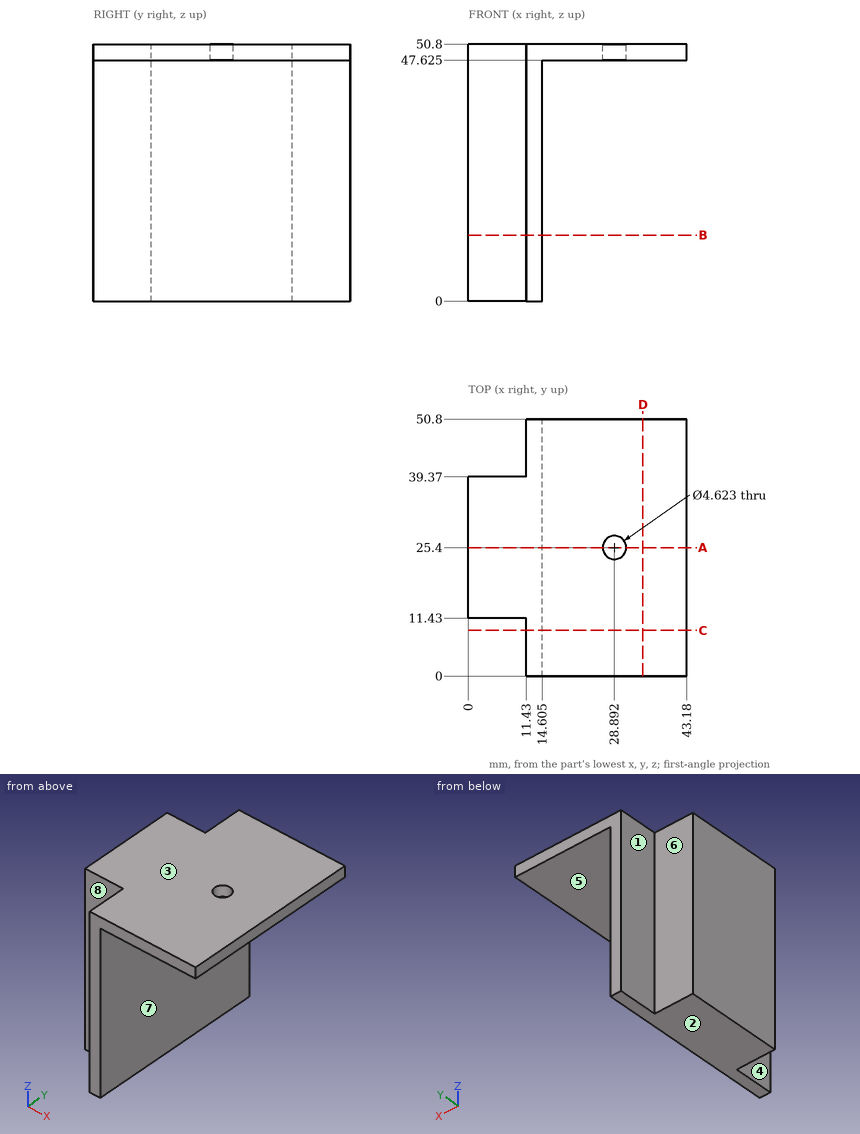
Job drawing, mm, ordinate dimensions from the low corner. One solid piece. A direction names the side the tool comes from. Round coordinates to 2 decimals unless told otherwise and drop trailing zeros. Loops run counter-clockwise (first coordinate to the right, second up) from the corner with the lowest first, then second, coordinate; pieces in that order, holes last. Notation, with made-up numbers: (85, -2) -> (142, -2) arc R22 ccw to (142, 16) -> close; hole circle Ø2 at (-7.75, 9.25). An arc over 180 degrees is marked (long way). Use a Markdown table: item, result.
1) Cut at B-B, the plane z = 13. List the corners of the cut face in (x, y) (1 decimal), and give its area (3 significant figures).
The answers:
| item | result |
|---|---|
| outline | (0, 11.4) -> (11.4, 11.4) -> (11.4, 0) -> (14.6, 0) -> (14.6, 50.8) -> (11.4, 50.8) -> (11.4, 39.4) -> (0, 39.4) -> close |
| area | 481 mm2 |
2) Pull direction Y, two halves, no side cores. Call the marked faces 6, 7 and 8: pulls with the +Y half, pulls with the -Y half, needs draft (parallel to the pull), parting line crosses it, or undercut.
The answers:
| item | result |
|---|---|
| face 6 | pulls with the +Y half |
| face 7 | needs draft |
| face 8 | pulls with the -Y half |
3) Cut at D-D, the plane x = 34.5. List the corners of the cut face in (y, z) (1 decimal), and give its area (3 significant figures).
The answers:
| item | result |
|---|---|
| outline | (0, 47.6) -> (50.8, 47.6) -> (50.8, 50.8) -> (0, 50.8) -> close |
| area | 161 mm2 |
4) Tool access for the marked faces 1, 2, 3, 4 and 5: list every direction of +Z, -Z, +X, -X, +Y, -Y with a clear straight run to the whole face (end or side of a thin tool).
The answers:
| item | result |
|---|---|
| face 1 | +Z, -Z, -X, +Y |
| face 2 | -Z, +X, -X, +Y, -Y |
| face 3 | +Z, +X, -X, +Y, -Y |
| face 4 | +Z, -Z, -X, -Y |
| face 5 | -Z, +X, +Y, -Y |
5) Drop flat-ended pins along their axis: pin 1 Ø5.5 at (x, z) = (5, 35.5) entering from -Y; pin 2 Ø5 at (y, z) = (15.5, 17.5) entering from +X (1 decimal); pin 3 Ø12.5 at (y, z) = (47.5, 15.5) entering from -X. Give the stop position or say it passes through.
The answers:
| item | result |
|---|---|
| pin 1 | stops at y = 11.43 |
| pin 2 | stops at x = 14.6 |
| pin 3 | stops at x = 11.43 |
6) Probe line 1 (Z direction, x = 36, y = 3.5) (1 decimal); line 2 (X direction, y = 48.5, z = 19) (1 decimal); line 3 (Y direction, x = 7, z = 15). List the from-to ranges inside material, lowest first. Write a range as [from, to].
The answers:
| item | result |
|---|---|
| line 1 | z = [47.6, 50.8] |
| line 2 | x = [11.4, 14.6] |
| line 3 | y = [11.43, 39.37] |
7) Cut at C-C, the plane y = 9. List the corners of the cut face in (x, z) (1 decimal).
The answers:
| item | result |
|---|---|
| outline | (11.4, 0) -> (14.6, 0) -> (14.6, 47.6) -> (43.2, 47.6) -> (43.2, 50.8) -> (11.4, 50.8) -> close |
8) Cut at A-A, the plane y = 25.4. List the corners of the cut face in (x, z) (1 decimal).
The answers:
| item | result |
|---|---|
| outline | (0, 0) -> (14.6, 0) -> (14.6, 47.6) -> (26.6, 47.6) -> (26.6, 50.8) -> (0, 50.8) -> close; (31.2, 47.6) -> (43.2, 47.6) -> (43.2, 50.8) -> (31.2, 50.8) -> close |
